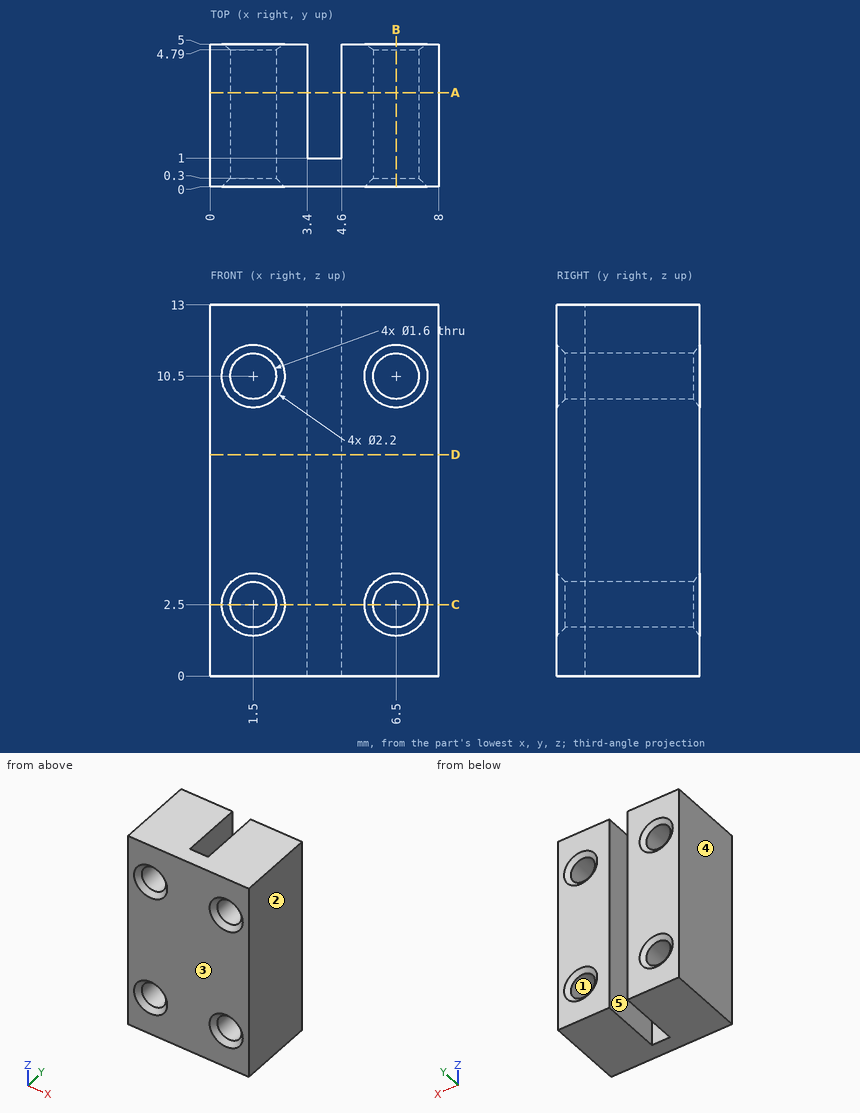
Can you work these out from the drawing? Everything is in mm from the part's minimum corner. A direction names the side the tool comes from. Round coordinates to 2 decimals unless told otherwise and drop trailing zeros. Write each loop counter-clockwise with the first axis right and the second up, starting at its lowest first coordinate (ties: lowest second). Pieces come first, ordered by that corner, then holes.
1. Suppose I cut it at C-C (z = 2.5). List the corners of the cut face in (x, y) for me, and give its area (3 significant figures).
2. Will these pins go through, and if not, where does the flat tip stop? pin 1 Ø1 at (x, z) = (4, 6) entering from +Y; pin 2 Ø1.8 at (x, z) = (6.5, 2.5) entering from -Y.
3. Suppose I cut it at A-A (y = 3.3). List the corners of the cut face in (x, z) for me.
4. Suppose I cut it at D-D (z = 7.75). List the corners of the cut face in (x, y) for me.
5. For the marked faces 4 and 5, which set-ups out of +Z, -Z, +X, -X, +Y, -Y let a thin tool reach every point of the face, with its end or its side?
6. I need wall thicknesses on L1, parallel to Z at x = 6.5, y = 3.6; L2, parallel to X at y = 3.6, z = 12.25; L3, parallel to X at y = 3.9, z = 10.5. Which ranges of each line are inside material? Lowest first, please.
7. Suppose I cut it at B-B (x = 6.5). List the corners of the cut face in (y, z) for me, and give its area (3 significant figures).
8. If we mould it in two halves opening along X, with no side actions, what happens to the marked faces 1, 2 and 3? For each: released by +X, released by -X, zero draft, split by the parting line, or undercut.
Answer sheet:
1. outline: (0, 0) - (0.4, 0) - (0.7, 0.3) - (0.7, 4.79) - (0.4, 5) - (0, 5) - close; (2.3, 0.3) - (2.6, 0) - (5.4, 0) - (5.7, 0.3) - (5.7, 4.79) - (5.4, 5) - (4.6, 5) - (4.6, 1) - (3.4, 1) - (3.4, 5) - (2.6, 5) - (2.3, 4.79) - close; (7.3, 0.3) - (7.6, 0) - (8, 0) - (8, 5) - (7.6, 5) - (7.3, 4.79) - close
1. area: 18.9 mm2
2. pin 1: stops at y = 1
2. pin 2: stops at y = 0.2
3. outline: (0, 0) - (3.4, 0) - (3.4, 13) - (0, 13) - close; (4.6, 0) - (8, 0) - (8, 13) - (4.6, 13) - close; hole circle Ø1.6 at (1.5, 2.5); hole circle Ø1.6 at (1.5, 10.5); hole circle Ø1.6 at (6.5, 2.5); hole circle Ø1.6 at (6.5, 10.5)
4. outline: (0, 0) - (8, 0) - (8, 5) - (4.6, 5) - (4.6, 1) - (3.4, 1) - (3.4, 5) - (0, 5) - close
5. face 4: +Z, -Z, -X, +Y, -Y
5. face 5: +Z, -Z, +Y
6. L1: z = 0 to 1.7, 3.3 to 9.7, 11.3 to 13
6. L2: x = 0 to 3.4, 4.6 to 8
6. L3: x = 0 to 0.7, 2.3 to 3.4, 4.6 to 5.7, 7.3 to 8
7. outline: (0, 0) - (5, 0) - (5, 1.4) - (4.79, 1.7) - (0.3, 1.7) - (0, 1.4) - close; (0, 3.6) - (0.3, 3.3) - (4.79, 3.3) - (5, 3.6) - (5, 9.4) - (4.79, 9.7) - (0.3, 9.7) - (0, 9.4) - close; (0, 11.6) - (0.3, 11.3) - (4.79, 11.3) - (5, 11.6) - (5, 13) - (0, 13) - close
7. area: 48.7 mm2
8. face 1: undercut
8. face 2: released by +X
8. face 3: zero draft
